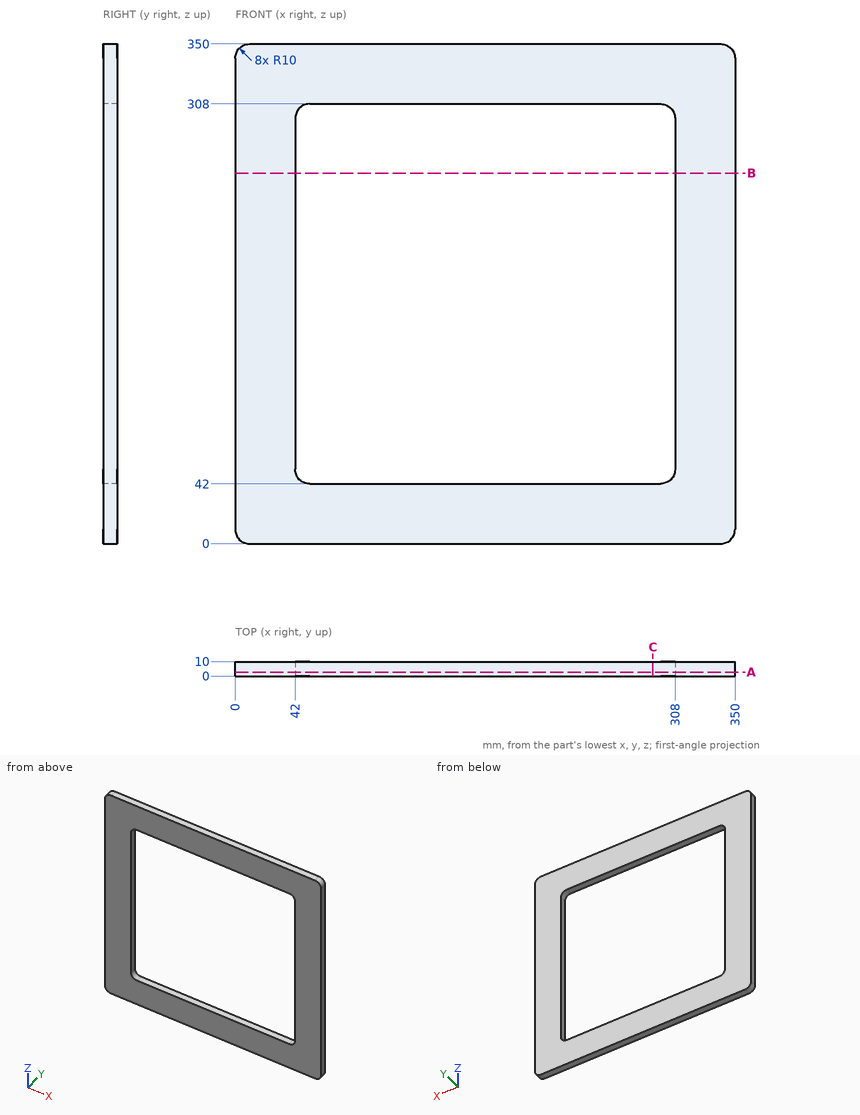
The drawing under review shows one solid part. Ordinate dimensions are in mm from its lowest x, y, z. Round coordinates to 2 decimals unless told otherwise and drop trailing zeros. Loops run counter-clockwise (first coordinate to the right, second up) from the corner with the lowest first, then second, coordinate; pieces in that order, holes last. Notation, with made-up numbers: (84, 11) - (110, 11) arc R17 ccw to (110, 38) - close; hole circle Ø6 at (52, 1). An arc over 180 degrees is marked (long way). One line per item, written item: value. Start each with the question number.
1) Consider section C-C on x = 292.5. Give the boundary of the cut face in (y, z).
2) To check wall thickness, follow L1, parallel to X at y = 9.25, z = 219; L2, parallel to X at y = 2, z = 306. State the ranges of each line that lie inside material, in increasing order. Write a range as from..to.
3) Consider section A-A on y = 2.75. Give the boundary of the cut face in (x, z).
4) Consider section B-B on z = 259.5. Give the boundary of the cut face in (x, y).
Reported:
1. outline: (0, 0) - (10, 0) - (10, 42) - (0, 42) - close; (0, 308) - (10, 308) - (10, 350) - (0, 350) - close
2. L1: x = 0..42, 308..350
2. L2: x = 0..46, 304..350
3. outline: (0, 10) arc R10 ccw to (10, 0) - (340, 0) arc R10 ccw to (350, 10) - (350, 340) arc R10 ccw to (340, 350) - (10, 350) arc R10 ccw to (0, 340) - close; hole (42, 52) arc R10 ccw to (52, 42) - (298, 42) arc R10 ccw to (308, 52) - (308, 298) arc R10 ccw to (298, 308) - (52, 308) arc R10 ccw to (42, 298) - close
4. outline: (0, 0) - (42, 0) - (42, 10) - (0, 10) - close; (308, 0) - (350, 0) - (350, 10) - (308, 10) - close
